Verification items for the finished model (mm, model axes). Face numbers are marked on the shaded views. A direction names the side the tool comes from. Give positions to 0.01 mm unless a question says otherwise; leave off trailing zeros. Loops run counter-clockwise (first coordinate to the right, second up) from the corner with the lowest first, then second, coordinate; pieces in that order, holes last. Notation, with made-up numbers: (-6.75, 40.5) - (38.25, 40.5) arc R25 cw to (38.25, 79.5) - close; hole circle Ø4 at (45, 42.5). An arc over 180 degrees is marked (long way). Use one line per item in the form item = value.
```python
from build123d import *

# Parameters (mm, degrees)
BOSS_EXTRUDE1_DEPTH  = 3.81
SKETCH3_W            = 12.7
SKETCH3_H            = 4
SKETCH3_W_2          = 4
SKETCH3_H_2          = 12.7
BOSS_EXTRUDE2_DEPTH  = 2.54
M2_CLEARANCE_HOLE1_D = 2.4
M2_CLEARANCE_HOLE2_D = 2.4


with BuildPart() as part:
    # Sketch2 → Boss-Extrude1 (new body, symmetric)
    with BuildSketch(Plane(origin=(0, 0, 0), x_dir=(1, 0, 0), z_dir=(0, 1, 0))):
        with BuildLine():
            Line((-3.746, 20.86), (0.254, 20.86))
            Line((0.254, 20.86), (0.254, 8.16))
            Line((0.254, 8.16), (-0.246, 8.16))
            ThreePointArc((-0.246, 8.16), (1.862831175, 3.068831175), (6.954, 0.96))
            Line((6.954, 0.96), (6.954, 1.46))
            Line((6.954, 1.46), (19.654, 1.46))
            Line((19.654, 1.46), (19.654, -2.54))
            Line((19.654, -2.54), (6.954, -2.54))
            Line((6.954, -2.54), (6.954, -2.04))
            ThreePointArc((6.954, -2.04), (-0.258489168, 0.947510832), (-3.246, 8.16))
            Line((-3.246, 8.16), (-3.746, 8.16))
            Line((-3.746, 8.16), (-3.746, 20.86))
        make_face()
    extrude(amount=BOSS_EXTRUDE1_DEPTH, both=True)

    # Sketch3 → Boss-Extrude2 (add)
    with BuildSketch(Plane(origin=(0, 3.81, 0), x_dir=(1, 0, 0), z_dir=(0, 1, 0))):
        with Locations((13.304, -0.54)):
            Rectangle(SKETCH3_W, SKETCH3_H)
        with Locations((-1.746, 14.51)):
            Rectangle(SKETCH3_W_2, SKETCH3_H_2)
    boss_extrude2 = extrude(amount=BOSS_EXTRUDE2_DEPTH)

    # Mirror1: Boss-Extrude2 across plane
    add(boss_extrude2.mirror(Plane.ZX))

    # M2 Clearance Hole1 (through all)
    with Locations(Plane(origin=(0.254, 0, 0), x_dir=(0, 0, -1), z_dir=(1, 0, 0))):
        with Locations((14.51, 3.175), (14.51, -3.175)):
            Hole(M2_CLEARANCE_HOLE1_D / 2)

    # M2 Clearance Hole2 (through all)
    with Locations(Plane(origin=(0, 0, -1.46), x_dir=(-1, 0, 0), z_dir=(0, 0, -1))):
        with Locations((-13.304, 3.175), (-13.304, -3.175)):
            Hole(M2_CLEARANCE_HOLE2_D / 2)


solid = part.part
```
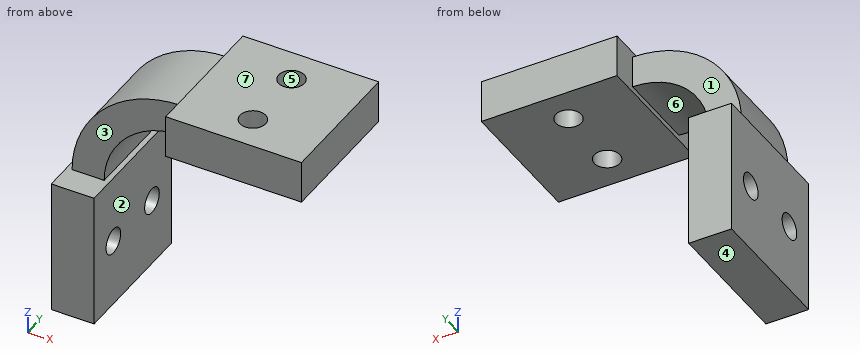
1. Section check D-D, the plane x = -2. Record the cut outline in (y, z) (3 decimals).
Result set:
outline = (-6.35, -20.86) - (6.35, -20.86) - (6.35, -8.16) - (3.81, -8.16) - (3.81, -3.275) - (-3.81, -3.275) - (-3.81, -8.16) - (-6.35, -8.16) - close; hole circle Ø2.4 at (-3.175, -14.51); hole circle Ø2.4 at (3.175, -14.51)
2. Section check B-B, the plane z = -14.51. Record the cut outline in (x, y) (3 decimals), then the cut area to 3 significant figures.
Result set:
outline = (-3.746, -6.35) - (0.254, -6.35) - (0.254, -4.375) - (-3.746, -4.375) - close; (-3.746, -1.975) - (0.254, -1.975) - (0.254, 1.975) - (-3.746, 1.975) - close; (-3.746, 4.375) - (0.254, 4.375) - (0.254, 6.35) - (-3.746, 6.35) - close
area = 31.6 mm²
3. Depth check by flat-ended pin: pin 1 Ø4 at (y, z) = (2.5, -14) entering from +X; pin 2 Ø11 at (x, z) = (0, -1.5) entering from -Y; pin 3 Ø4 at (x, y) = (6.5, 2) entering from -Z. Enter the tip coordinate at first touch or a pass-through.
Result set:
pin_1 = 0.25
pin_2 = -3.81
pin_3 = -1.46
4. Section check A-A, the plane y = -5.25. Record the cut outline in (x, z).
Result set:
outline = (-3.75, -20.86) - (0.25, -20.86) - (0.25, -8.16) - (-3.75, -8.16) - close; (6.95, -1.46) - (19.65, -1.46) - (19.65, 2.54) - (6.95, 2.54) - close
5. Scan lines: probe 1 along Y at (x, z) = (-2.45, -14.51) (3 decimals); probe 2 along X at (y, z) = (-2, -18.25); probe 3 along Z at (x, y) = (-1.5, 3). Record each from-to range of solid material in increasing order.
Result set:
probe_1 = -6.35 to -4.375, -1.975 to 1.975, 4.375 to 6.35
probe_2 = -3.75 to 0.25
probe_3 = -20.86 to -15.7, -13.32 to -2.45
6. Section check C-C, the plane y = 1.5. Record the cut outline in (x, z), then the cut area to 3 significant figures.
Result set:
outline = (-3.75, -20.86) - (0.25, -20.86) - (0.25, -8.16) - (-0.25, -8.16) arc R7.2 cw to (6.95, -0.96) - (6.95, -1.46) - (19.65, -1.46) - (19.65, 2.54) - (6.95, 2.54) - (6.95, 2.04) arc R10.2 ccw to (-3.25, -8.16) - (-3.75, -8.16) - close
area = 143 mm²
7. Draft check along Z on the marked faces 4, 5, 6 and 7. Enter one of: released by +Z, released by -Z, zero draft, split by the parting line, or undercut.
Result set:
face_4 = released by -Z
face_5 = zero draft
face_6 = undercut
face_7 = released by +Z
8. Tool access check on the marked faces 1, 2 and 3. Record the directions out of +Z, -Z, +X, -X, +Y, -Y that give a thin tool (end or side, any length) a straight path to the whole face; none if there is none.
Result set:
face_1 = +Z, -X, +Y
face_2 = -Z, +X, +Y, -Y
face_3 = +Z, -X, -Y
